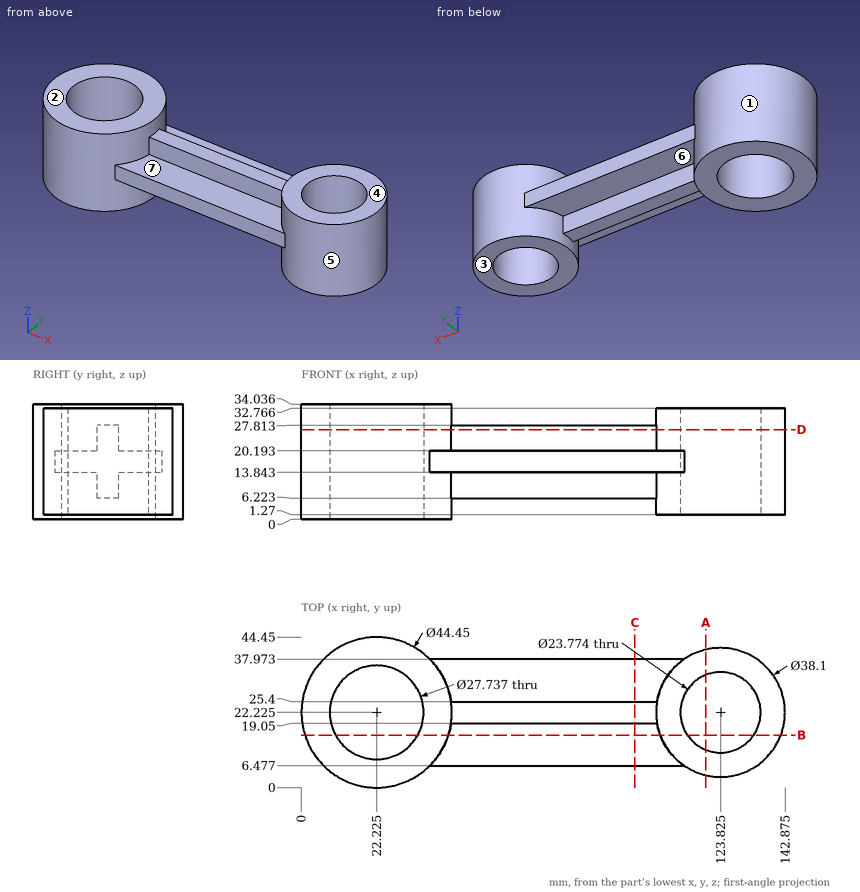
For this review, use the dimensioned drawing (mm, ordinates from the lowest corner) and the shaded views. A direction names the side the tool comes from. Round coordinates to 2 decimals unless told otherwise and drop trailing zeros. Write each loop counter-clockwise with the first axis right and the second up, starting at its lowest first coordinate (ties: lowest second). Pieces come first, ordered by that corner, then holes. Notation, with made-up numbers: M 58,-23 L 81,-23 A18 ccw 81,-4 Z; hole C -34,37.5 d10. An arc over 180 degrees is marked long. Use CSV: the item, a comma, the result in double quotes. Start each with the question number.
(1) Tool access review of the marked faces 3, 4, 5, 6 and 7: name each direction out of +Z, -Z, +X, -X, +Y, -Y from which nothing blocks a thin tool from reaching the whole face with its end or side.
(2) We need section A-A, the plane x = 119.5. State the section outline as (y, z) points, then the cut area to 3 significant figures.
(3) We need section D-D, the plane z = 26.5. State how many separate pieces and enclosed holes the cut face has, then the cut area to 3 significant figures.
(4) Clearance check with flat-ended pins moving along their axes: P1, Ø8.5, axis at x = 65.5, z = 22.5, coming from the +Y side; P2, Ø12, axis at y = 11.5, z = 10, coming from the +X side; P3, Ø4, axis at y = 32, z = 8.5, coming from the +X side. State where each tip first meets the part, or that it passes through.
(5) We need section C-C, the plane x = 98.5. State the section outline as (y, z) points, then the cut area to 3 significant figures.
(6) The part is to be moulded in two halves that separate along X. For the marked faces 1 and 2, say which applies: +X half, -X half, draft (parallel to the pull), parting line (faces both ways), or undercut.
(7) We need section B-B, the plane y = 15.5. State the section outline as (x, z) points.
(8) For line 1 along X through (y, z) = (21.5, 25) (1 decimal); line 2 along X through (y, z) = (25, 2) (1 decimal); line 3 along X through (y, z) = (17.5, 19.5) (1 decimal), list the stretches that pass through material, from the lowest coordinate up.
Findings:
1,face 3,"-Z, +X, +Y, -Y"
1,face 4,"+Z, +X, +Y, -Y"
1,face 5,"none"
1,face 6,"-Z, +Y"
1,face 7,"+Z, -Y"
2,outline,"M 3.67,1.27 L 11.15,1.27 L 11.15,32.77 L 3.67,32.77 Z; M 33.3,1.27 L 40.78,1.27 L 40.78,32.77 L 33.3,32.77 Z"
2,area,"471 mm^2"
3,separate pieces,"1"
3,enclosed holes,"2"
3,area,"2,030 mm^2"
4,P1,"y = 37.97"
4,P2,"x = 142.28"
4,P3,"x = 141.22"
5,outline,"M 6.48,13.84 L 19.05,13.84 L 19.05,6.22 L 25.4,6.22 L 25.4,13.84 L 37.97,13.84 L 37.97,20.19 L 25.4,20.19 L 25.4,27.81 L 19.05,27.81 L 19.05,20.19 L 6.48,20.19 Z"
5,area,"297 mm^2"
6,face 1,"undercut"
6,face 2,"draft"
7,outline,"M 1.04,0 L 10.1,0 L 10.1,34.04 L 1.04,34.04 Z; M 34.35,0 L 43.41,0 L 43.41,13.84 L 106,13.84 L 106,1.27 L 114.02,1.27 L 114.02,32.77 L 106,32.77 L 106,20.19 L 43.41,20.19 L 43.41,34.04 L 34.35,34.04 Z; M 133.63,1.27 L 141.65,1.27 L 141.65,32.77 L 133.63,32.77 Z"
8,line 1,"0 to 8.4, 36.1 to 112, 135.7 to 142.9"
8,line 2,"0.2 to 8.6, 35.8 to 44.3, 105 to 112.3, 135.4 to 142.7"
8,line 3,"0.5 to 9.2, 35.3 to 112.9, 134.7 to 142.3"
